Verification items for the finished model (mm, model axes). A direction names the side the tool comes from. Round coordinates to 2 decimals unless told otherwise and drop trailing zeros. Order: outer loops, then holes, each group sorted by start corner. A loop starts at its lowest first (then second) coordinate and runs counter-clockwise, first axis right, second up. Notation, with made-up numbers: (-17.5, 3) -> (24.5, 3) arc R33 ccw to (24.5, 42) -> close; hole circle Ø11 at (67, 16). An arc over 180 degrees is marked (long way). Answer in a Markdown table with one row per item. Add a question column.
```python
from build123d import *

# Parameters (mm, degrees)
F2_R     = 150
F2_R_2   = 2.2
F2_R_3   = 10
F2_R_4   = 5.25
F3_DEPTH = 15
F4_DEPTH = 8


with BuildPart() as f3:
    # F2 (on Right) → F3 (new body)
    with BuildSketch(Plane.YZ):
        Circle(F2_R)
        with Locations((0, -15)):
            Circle(F2_R_2, mode=Mode.SUBTRACT)
        with Locations((-20, 0)):
            Circle(F2_R_2, mode=Mode.SUBTRACT)
        Circle(F2_R_3, mode=Mode.SUBTRACT)
        with Locations((0, 15)):
            Circle(F2_R_2, mode=Mode.SUBTRACT)
        with Locations((20, 0)):
            Circle(F2_R_2, mode=Mode.SUBTRACT)
        Circle(F2_R_3)
        Circle(F2_R_4, mode=Mode.SUBTRACT)
    extrude(amount=-F3_DEPTH)

    # F2 (on Right) → F4 (cut)
    with BuildSketch(Plane.YZ):
        Circle(F2_R_3)
        Circle(F2_R_4, mode=Mode.SUBTRACT)
    extrude(amount=-F4_DEPTH, mode=Mode.SUBTRACT)


solid = f3.part
```
1) Thickness scan on L1, parallel to Z at x = -7.25, y = 0; L2, parallel to Z at x = -5.25, y = 20; L3, parallel to X at y = 8.5, z = 0.5. Record the ranges inside material, lowest first. Write a range as [from, to].
2) Cross-section at A-A, the plane y = -27. Record the boundary of the cut face in (x, z).
3) Tool access check on faces 1 (the face through (-3.94, -2.17, -9.76)), 2 (the face through (-15, 31, 2)). Record the directions out of +Z, -Z, +X, -X, +Y, -Y that give a thin tool (end or side, any length) a straight path to the whole face; none if there is none.
4) Draft check along Y on faces 3 (the face through (0, 31, 2)), 4 (the face through (-8, 4, -4)), 5 (the face through (-11.5, 5, 1.6)), 6 (the face through (-7.395, -19.527, 148.724)). Enter one of: +Y half, -Y half, draft (parallel to the pull), parting line (faces both ways), or undercut.
5) Depth check by flat-ended pin: P1, Ø5, axis at x = -4.5, z = -89.5, coming from the -Y side; P2, Ø3, axis at x = -6.5, z = 27.5, coming from the -Y side; P3, Ø1.5, axis at x = -8.5, y = -63, coming from the +Z side. Enter the tip coordinate at first touch or a pass-through.
6) Cross-section at B-B, the plane z = -66. Record the boundary of the cut face in (x, y), and give its area (3 significant figures).
Results below:
| question | item | result |
|---|---|---|
| 1 | L1 | [-150, -17.2], [-12.8, -10], [10, 12.8], [17.2, 150] |
| 1 | L2 | [-148.66, -2.2], [2.2, 148.66] |
| 1 | L3 | [-15, -8] |
| 2 | outline | (-15, -147.55) -> (0, -147.55) -> (0, 147.55) -> (-15, 147.55) -> close |
| 3 | face 1 | +X |
| 3 | face 2 | +Z, -Z, -X, +Y, -Y |
| 4 | face 3 | draft |
| 4 | face 4 | undercut |
| 4 | face 5 | undercut |
| 4 | face 6 | parting line |
| 5 | P1 | y = -122.19 |
| 5 | P2 | y = -147.73 |
| 5 | P3 | z = 136.47 |
| 6 | outline | (-15, -134.7) -> (0, -134.7) -> (0, 134.7) -> (-15, 134.7) -> close |
| 6 | area | 4,040 mm² |
